Work out the finished part from the listing and answer in its coordinate system (mm). A direction names the side the tool comes from. Coordinates: 2 decimals unless noted, no trailing zeros. Loops run counter-clockwise (first coordinate to the right, second up) from the corner with the lowest first, then second, coordinate; pieces in that order, holes last. Notation, with made-up numbers: (19, 53.25) -> (73, 53.25) arc R11 cw to (73, 71.25) -> close; hole circle Ø10 at (30.25, 77). An arc over 180 degrees is marked (long way). One line per question, with ' | ' between items.
```python
from build123d import *

# Parameters (mm, degrees)
F0_W      = 90
F0_H      = 60
F1_DEPTH  = 25
F1_FACE_W = 90
F1_FACE_H = 60
F2_DEPTH  = 60
F4_DEPTH  = 25


with BuildPart() as f1:
    # F0 (on Front) → F1 (new body)
    with BuildSketch(Plane.XZ):
        with Locations((45, 30)):
            Rectangle(F0_W, F0_H)
    extrude(amount=F1_DEPTH)

    # F1_face (on face) → F2 (join)
    with BuildSketch(Plane(origin=(45, -25, 30), x_dir=(1, 0, 0), z_dir=(0, -1, 0))):
        Rectangle(F1_FACE_W, F1_FACE_H)
    extrude(amount=F2_DEPTH)

    # F3 (on face) → F4 (join)
    with BuildSketch(Plane.YZ.offset(90)):
        Polygon((0, 7.243759), (0, 60), (-10.070629, 7.243759), align=None)
    extrude(amount=F4_DEPTH)


solid = f1.part
```
1) Find section A-A (x = 106.5). Write down the section's boundary in (y, z), plus the area to 3 significant figures.
Check values:
outline: (-10.07, 7.24) -> (0, 7.24) -> (0, 60) -> close | area: 266 mm^2
2) Find section B-B (z = 42.5). Write down the section's boundary in (x, y).
Check values:
outline: (0, -85) -> (90, -85) -> (90, -3.34) -> (115, -3.34) -> (115, 0) -> (0, 0) -> close
3) Find section C-C (y = -7). Write down the section's boundary in (x, z), plus the area to 3 significant figures.
Check values:
outline: (0, 0) -> (90, 0) -> (90, 7.24) -> (115, 7.24) -> (115, 23.33) -> (90, 23.33) -> (90, 60) -> (0, 60) -> close | area: 5,800 mm^2
4) Flat-ended cylindrical pins translate along their axes: pin 1 (2 mm diameter, centred on x = 69, z = 49.5, fed in from +Y); pin 2 (5 mm diameter, centred on x = 94, z = 52.5, fed in from -Y); pin 3 (3 mm diameter, centred on x = 102, y = -3.5, fed in from -Z); pin 4 (1 mm diameter, centred on y = -33, z = 19.5, fed in from +X). Find the tip coordinate at first contact, or state that the pin passes through.
Check values:
pin 1: stops at y = 0 | pin 2: stops at y = -1.91 | pin 3: stops at z = 7.24 | pin 4: stops at x = 90
5) For faces 1 (the face through (102.325, -4.965, 33.991)), 2 (the face through (115, -3, 22)), 3 (the face through (102, -5, 7.244)), determine the directions among +Z, -Z, +X, -X, +Y, -Y from which every point of the face is accessible in a straight line to the end or side of a thin tool.
Check values:
face 1: +Z, +X, -Y | face 2: +Z, -Z, +X, +Y, -Y | face 3: -Z, +X, +Y, -Y
6) Find section D-D (y = -42). Write down the section's boundary in (x, z), plus the area to 3 significant figures.
Check values:
outline: (0, 0) -> (90, 0) -> (90, 60) -> (0, 60) -> close | area: 5,400 mm^2
7) Find the intervals of material crossed by line 1 along X through (y, z) = (-64.5, 31); line 2 along Y through (x, z) = (91, 48.5); line 3 along Y through (x, z) = (107.5, 56), in increasing order.
Check values:
line 1: x = 0 to 90 | line 2: y = -2.2 to 0 | line 3: y = -0.76 to 0
